For this review, take the finished solid that the model builds, in its own axes (mm). Give positions to 0.01 mm unless a question says otherwise; leave off trailing zeros. Loops run counter-clockwise (first coordinate to the right, second up) from the corner with the lowest first, then second, coordinate; pieces in that order, holes last. Notation, with made-up numbers: M 41.25,-20.75 L 67.25,-20.75 A25 ccw 67.25,15.25 Z; hole C 19.25,71.25 d7. An arc over 180 degrees is marked long. Use CSV: the item, a comma, the result in double quotes. Start each with the question number.
1. Take a section at B-B, the plane x = -39.5. Write out the cut boundary in (y, z), and give its area (3 significant figures).
2. To check wall thickness, follow line 1 (X direction, y = 82, z = 3); line 2 (X direction, y = 98, z = 1.25); line 3 (Y direction, x = -40, z = 1.75). State the ranges of each line that lie inside material, in increasing order. Write a range as [from, to].
3. Take a section at C-C, the plane y = 75. Write out the cut boundary in (x, z).
4. Insertion check: P1, Ø1.9, axis at x = 41.5, z = 2, coming from the +Y side; P2, Ø1.9, axis at y = 23, z = 4.5, coming from the +X side; P3, Ø3, axis at x = 2, z = 1.5, coming from the -Y side. Each pin has a flat end and moves straight along its axis. Give the tip position at first contact, or say it passes through.
Autodesk Inventor part; units mm, degrees
ref_plane "YZ Plane" through (0, 0, 0) normal (1, 0, 0) x (0, 1, 0)
ref_plane "XZ Plane" through (0, 0, 0) normal (0, 1, 0) x (-1, 0, 0)
ref_plane "XY Plane" through (0, 0, 0) normal (0, 0, 1) x (1, 0, 0)
sketch "Sketch1" plane through (0, 0, 0) normal (0, 0, 1) x (1, 0, 0)
  line L0 (-51.6543, 109.7487) -> (38.1457, 109.7487) construction
  line L1 (38.1457, -13.2513) -> (-51.6543, -13.2513) construction
  line L2 (-51.6543, -13.2513) -> (-51.6543, 109.7487) construction
  line L3 (38.1457, 94.7487) -> (44.5457, 94.7487)
  line L4 (44.5457, 94.7487) -> (44.5457, 82.7487)
  line L5 (44.5457, 82.7487) -> (38.1457, 82.7487)
  line L6 (38.1457, 82.7487) -> (38.1457, 94.7487)
  line L7 (44.5457, 67.7487) -> (44.5457, 55.7487)
  line L8 (44.5457, 55.7487) -> (38.1457, 55.7487)
  line L9 (38.1457, 55.7487) -> (38.1457, 67.7487)
  line L10 (38.1457, 67.7487) -> (44.5457, 67.7487)
  line L11 (44.5457, 40.7487) -> (44.5457, 28.7487)
  line L12 (44.5457, 28.7487) -> (38.1457, 28.7487)
  line L13 (38.1457, 28.7487) -> (38.1457, 40.7487)
  line L14 (38.1457, 40.7487) -> (44.5457, 40.7487)
  line L15 (44.5457, 13.7487) -> (44.5457, 1.7487)
  line L16 (44.5457, 1.7487) -> (38.1457, 1.7487)
  line L17 (38.1457, 1.7487) -> (38.1457, 13.7487)
  line L18 (38.1457, 13.7487) -> (44.5457, 13.7487)
  line L19 (38.1457, 109.7487) -> (38.1457, -13.2513)
  line L20 (38.1457, -13.2513) -> (-51.6543, -13.2513)
  line L21 (11.1457, -13.2513) -> (23.1457, -13.2513)
  line L22 (23.1457, -13.2513) -> (23.1457, -19.6513)
  line L23 (23.1457, -19.6513) -> (11.1457, -19.6513)
  line L24 (11.1457, -19.6513) -> (11.1457, -13.2513)
  line L25 (-15.8543, -19.6513) -> (-15.8543, -13.2513)
  line L26 (-3.8543, -19.6513) -> (-15.8543, -19.6513)
  line L27 (-3.8543, -13.2513) -> (-3.8543, -19.6513)
  line L28 (-42.8543, -19.6513) -> (-42.8543, -13.2513)
  line L29 (-30.8543, -19.6513) -> (-42.8543, -19.6513)
  line L30 (-30.8543, -13.2513) -> (-30.8543, -19.6513)
  line L31 (-51.6543, -13.2513) -> (38.1457, 109.7487)
  point P0 (0, 0)
  dimension "d0" = 89.8
  dimension "d1" = 123
  dimension "d2" = 12
  dimension "d3" = 6.4
  dimension "d4" = 15
  dimension "d7" = 27
  dimension "d12" = 12
  dimension "d13" = 6.4
  dimension "d14" = 15
  dimension "d17" = 27
extrude "Extrusion1" add sketch "Sketch1" along normal blind 6.4
properties part number "mdf_support"
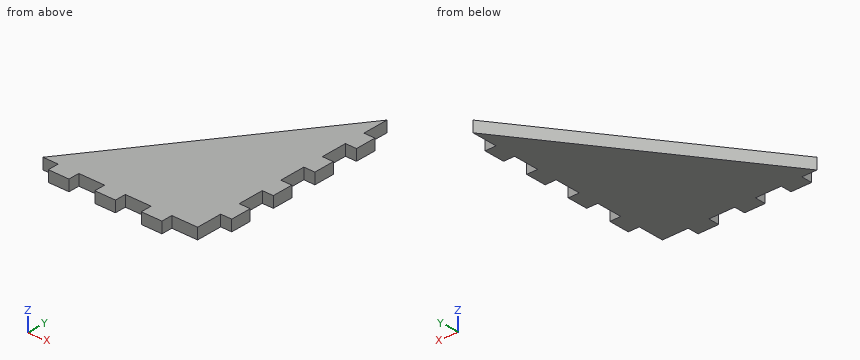
Result set:
1,outline,"M -19.65,0 L 3.4,0 L 3.4,6.4 L -19.65,6.4 Z"
1,area,"148 mm2"
2,line 1,"[17.89, 38.15]"
2,line 2,"[29.57, 38.15]"
2,line 3,"[-19.65, 2.71]"
3,outline,"M 12.78,0 L 38.15,0 L 38.15,6.4 L 12.78,6.4 Z"
4,P1,"y = 94.75"
4,P2,"x = 38.15"
4,P3,"y = -13.25"
